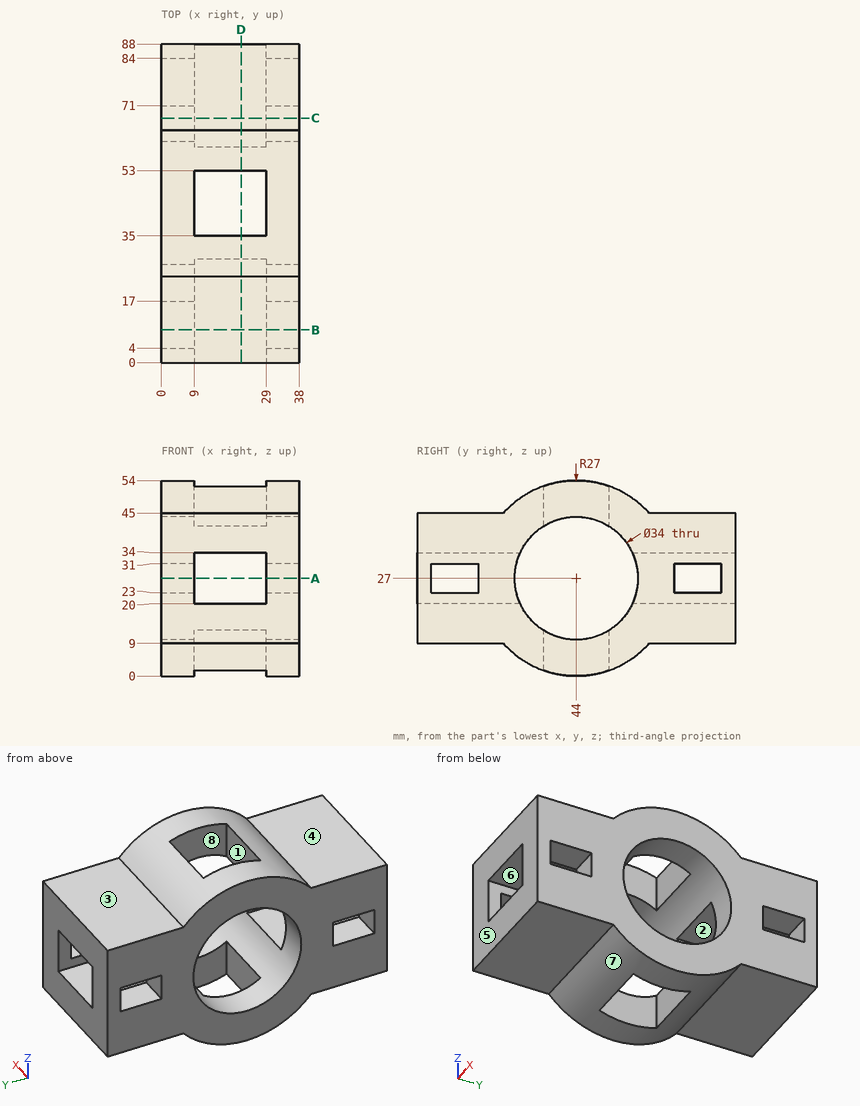
Drawing for the job (mm, zero at the part's lowest x, y, z). A direction names the side the tool comes from. Round coordinates to 2 decimals unless told otherwise and drop trailing zeros. Loops run counter-clockwise (first coordinate to the right, second up) from the corner with the lowest first, then second, coordinate; pieces in that order, holes last. Notation, with made-up numbers: (11.25, 72.25) - (70.25, 72.25) arc R21 cw to (70.25, 76.25) - close; hole circle Ø9 at (21.25, -36.75). An arc over 180 degrees is marked (long way). Return JSON: item names as keys, results as strings. Group by question number.
Q1. Flat gauge pins, fed straight in: pin 1 Ø10 at (x, y) = (6.5, 9) entering from -Z; pin 2 Ø5 at (x, y) = (27, 78) entering from +Z; pin 3 Ø5.5 at (x, z) = (19.5, 49) entering from -Y. Where does each tip first touch, or does it go through?
Q2. Band-saw the part on D-D on x = 22. Give the cut face in (y, z).
Q3. Band-saw the part on C-C on y = 67.5. Give the cut face in (x, z), plus the area to 3 significant figures.
Q4. Drill centre lines: line 1 along Z through (x, y) = (8.5, 44); line 2 along Y through (x, z) = (33.5, 26); line 3 along Y through (x, z) = (31.5, 23.5). Where is each one in solid material? Low to high. Write a range as [from, to].
Q5. Tool access for the marked faces 1, 2, 3 and 4: list every direction of +Z, -Z, +X, -X, +Y, -Y with a clear straight run to the whole face (end or side of a thin tool).
Q6. Band-saw the part on A-A on z = 27. Give the number of separate pieces and of enclosed holes in the cut face, plus the area to 3 significant figures.
Q7. Band-saw the part on B-B on y = 9. Give the cut face in (x, z), plus the area to 3 significant figures.
Q8. Two-plate mould, pull along Y, no slides. Class the marked faces 5, 6, 7 and 8: +Y half, -Y half, draft (parallel to the pull), parting line (faces both ways), or undercut.
Solutions:
{
 "1": {"pin 1": "stops at z = 9", "pin 2": "stops at z = 45", "pin 3": "stops at y = 25.07"},
 "2": {"outline": "(0, 9) - (23.88, 9) arc R27 ccw to (35, 1.54) - (35, 12.58) arc R17 cw to (28.51, 20) - (0, 20) - close; (0, 34) - (28.51, 34) arc R17 cw to (35, 41.42) - (35, 52.46) arc R27 ccw to (23.88, 45) - (0, 45) - close; (53, 1.54) arc R27 ccw to (64.12, 9) - (88, 9) - (88, 20) - (59.49, 20) arc R17 cw to (53, 12.58) - close; (53, 41.42) arc R17 cw to (59.49, 34) - (88, 34) - (88, 45) - (64.12, 45) arc R27 ccw to (53, 52.46) - close"},
 "3": {"outline": "(0, 9) - (38, 9) - (38, 45) - (0, 45) - close; hole (9, 20) - (29, 20) - (29, 34) - (9, 34) - close", "area": "1,090 mm^2"},
 "4": {"line 1": "z = [0, 10], [44, 54]", "line 2": "y = [0, 4], [17, 27.03], [60.97, 71], [84, 88]", "line 3": "y = [0, 4], [17, 27.36], [60.64, 71], [84, 88]"},
 "5": {"face 1": "+Z, -Z", "face 2": "+Y, -Y", "face 3": "+Z, +X, -X, +Y", "face 4": "+Z, +X, -X, -Y"},
 "6": {"separate pieces": "8", "enclosed holes": "0", "area": "504 mm^2"},
 "7": {"outline": "(0, 9) - (38, 9) - (38, 23) - (29, 23) - (29, 20) - (9, 20) - (9, 23) - (0, 23) - close; (0, 31) - (9, 31) - (9, 34) - (29, 34) - (29, 31) - (38, 31) - (38, 45) - (0, 45) - close", "area": "944 mm^2"},
 "8": {"face 5": "-Y half", "face 6": "draft", "face 7": "parting line", "face 8": "undercut"}
}
